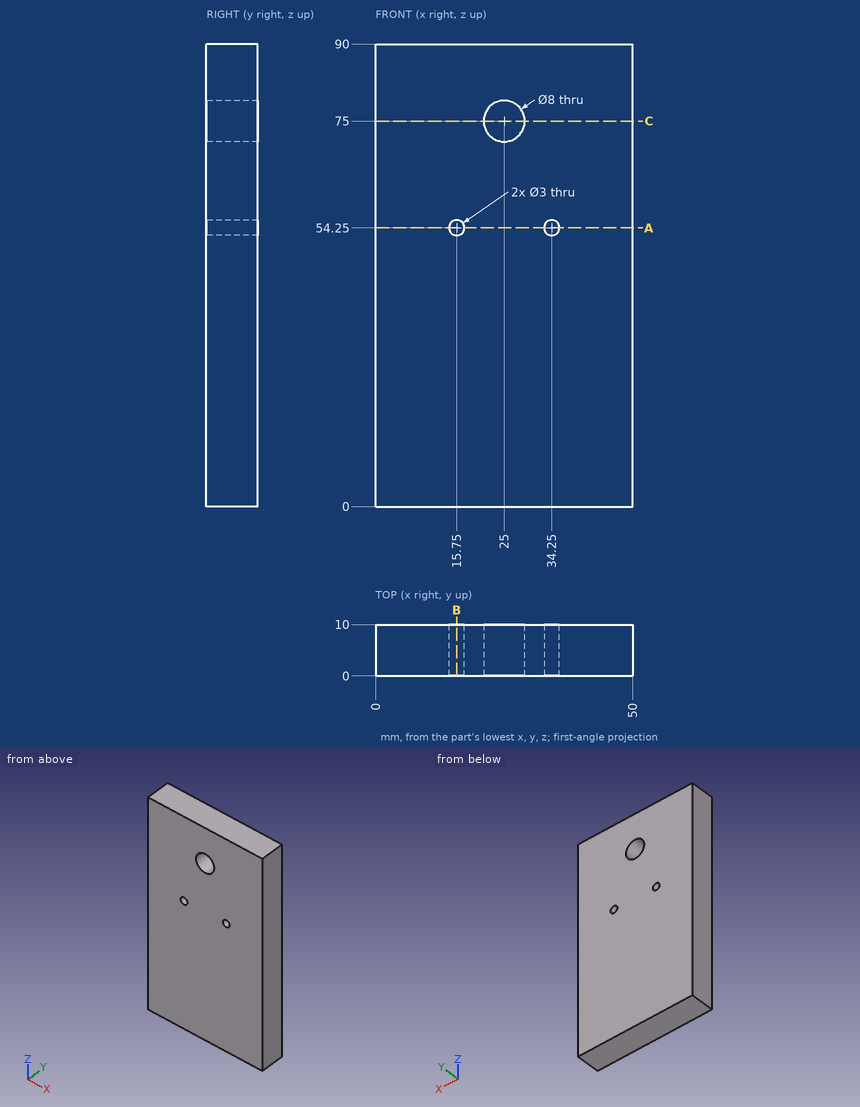
Verification items for this drawing (mm, ordinates from the low corner). Give positions to 0.01 mm unless a question says otherwise; leave off trailing zeros. Loops run counter-clockwise (first coordinate to the right, second up) from the corner with the lowest first, then second, coordinate; pieces in that order, holes last. Notation, with made-up numbers: M 52,78.25 L 97,78.25 A7 ccw 97,88.25 Z; hole C -30.75,-7 d6. An arc over 180 degrees is marked long. Answer as CSV lines item,"result".
Item 1: Depth check by flat-ended pin: P1, Ø2.5, axis at x = 34.25, z = 54.25, coming from the -Y side. Enter the tip coordinate at first touch or a pass-through.
Values:
P1,"passes through"
Item 2: Cross-section at C-C on z = 75. Record the cut outline in (x, y), and give its area (3 significant figures).
Values:
outline,"M 0,0 L 21,0 L 21,10 L 0,10 Z; M 29,0 L 50,0 L 50,10 L 29,10 Z"
area,"420 mm²"
Item 3: Material ranges on line 1 (Z direction, x = 25, y = 3.75); line 2 (Z direction, x = 34.25, y = 8.25); line 3 (X direction, y = 1, z = 78), recorded low to high.
Values:
line 1,"z = 0 to 71, 79 to 90"
line 2,"z = 0 to 52.75, 55.75 to 90"
line 3,"x = 0 to 22.35, 27.65 to 50"
Item 4: Cross-section at A-A on z = 54.25. Record the cut outline in (x, y), and give its area (3 significant figures).
Values:
outline,"M 0,0 L 14.25,0 L 14.25,10 L 0,10 Z; M 17.25,0 L 32.75,0 L 32.75,10 L 17.25,10 Z; M 35.75,0 L 50,0 L 50,10 L 35.75,10 Z"
area,"440 mm²"
Item 5: Cross-section at B-B on x = 15.75. Record the cut outline in (y, z), and give its area (3 significant figures).
Values:
outline,"M 0,0 L 10,0 L 10,52.75 L 0,52.75 Z; M 0,55.75 L 10,55.75 L 10,90 L 0,90 Z"
area,"870 mm²"
